Part model, mm, in its own coordinate system. Face numbers are marked on the shaded views. A direction names the side the tool comes from. Round coordinates to 2 decimals unless told otherwise and drop trailing zeros. Write each loop counter-clockwise with the first axis right and the second up, starting at its lowest first coordinate (ties: lowest second). Pieces come first, ordered by that corner, then holes. Notation, with made-up numbers: M 9.5,-0.5 L 48.5,-0.5 A12 cw 48.5,10.5 Z; hole C -22.5,81 d1. An arc over 180 degrees is marked long. Answer as a JSON object with one key per item and string values. Group by question number.
1. Drop flat-ended pins along their axis: pin 1 (12.5 mm diameter, centred on x = -46.71, z = 21.65, fed in from +Y); pin 2 (5 mm diameter, centred on y = -10.5, z = 29.5, fed in from +X); pin 3 (12.5 mm diameter, centred on x = 38.5, y = -14, fed in from +Z); pin 4 (1 mm diameter, centred on x = -34.5, z = 20, fed in from +Y). Give the stop position or say it passes through.
2. Which spindle directions (+Z, -Z, +X, -X, +Y, -Y) get a long thin tool onto all of the face, cutting with end or side? Do the marked faces 4 and 5. Say none if no direction does.
3. Two-plate mould, pull along Z, no slides. Class the marked faces 1, 2 and 3: +Z half, -Z half, draft (parallel to the pull), parting line (faces both ways), or undercut.
4. Band-saw the part on B-B, the plane x = -39. Write the cut outline in (y, z).
5. Band-saw the part on A-A, the plane z = 31. Write the cut outline in (x, y).
6. Band-saw the part on C-C, the plane y = -3. Write the cut outline in (x, z).
7. Band-saw the part on D-D, the plane x = 38. Write the cut outline in (y, z), plus the area to 3 significant figures.
8. Drill centre lines: line 1 (X direction, y = -8.75, z = 13); line 2 (X direction, y = -9.25, z = 15.5); line 3 (X direction, y = -4.5, z = 34). Where is each one in solid material? Low to high. Write a range as from..to.
from build123d import *

# Parameters (mm, degrees)
F0_R     = 10.5768156475
F1_DEPTH = 25.4
F2_R     = 5.8673814398
F3_DEPTH = 32.9165069776
F5_R     = 2.8308188493
F6_DEPTH = 16.9651473331


# Not quite as in the source:
# - a feature names something its author has since deleted; it is built from what else it names


with BuildPart() as f1:
    # F0 (on Front) → F1 (new body)
    with BuildSketch(Plane.XZ):
        Polygon((0, 38.612421602), (-61.9064718485, 38.612421602), (-61.9064718485, 5.6969146244), (1.8989704549, 5.6969146244), (65.7044127584, 12.2800152749), (65.7044127584, 22.1546681132), (65.7044127584, 22.6610619575), (0, 22.6610619575), align=None)
        with Locations((-46.7147007585, 21.6482765973)):
            Circle(F0_R, mode=Mode.SUBTRACT)
    extrude(amount=F1_DEPTH)

    # F2 (on face) → F3 (cut, through all)
    with BuildSketch(Plane.XY.offset(38.612421602)):
        with Locations((-18.1035287678, -13.1292007864)):
            Circle(F2_R)
    extrude(amount=-F3_DEPTH, mode=Mode.SUBTRACT)

    # F5 (on face) → F6 (cut, through all)
    with BuildSketch(Plane.XY.offset(22.6610619575)):
        with Locations((55.3233735263, -12.2800152749)):
            Circle(F5_R)
    extrude(amount=-F6_DEPTH, mode=Mode.SUBTRACT)


solid = f1.part
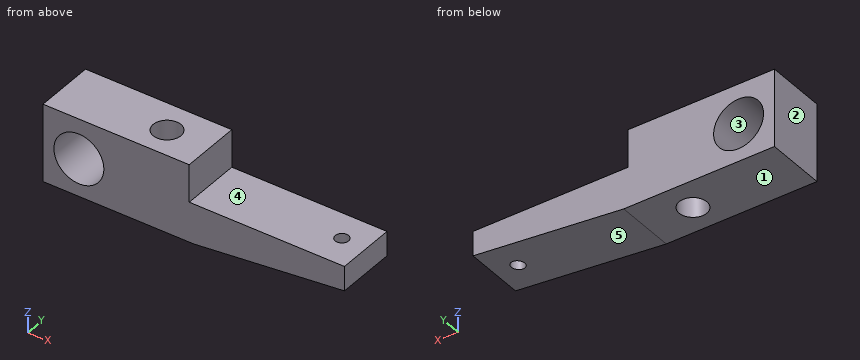
Worked answers:
{
 "1": {"pin 1": "passes through", "pin 2": "stops at x = 0", "pin 3": "stops at z = 22.66", "pin 4": "stops at y = 0"},
 "2": {"face 4": "+Z, +X, +Y, -Y", "face 5": "-Z, +X, +Y, -Y"},
 "3": {"face 1": "-Z half", "face 2": "draft", "face 3": "undercut"},
 "4": {"outline": "M -25.4,5.7 L 0,5.7 L 0,14.41 L -25.4,14.41 Z; M -25.4,28.88 L 0,28.88 L 0,38.61 L -25.4,38.61 Z"},
 "5": {"outline": "M -61.91,-25.4 L -51.66,-25.4 L -51.66,0 L -61.91,0 Z; M -41.77,-25.4 L 0,-25.4 L 0,0 L -41.77,0 Z; hole C -18.1,-13.13 d11.73"},
 "6": {"outline": "M -61.91,5.7 L 1.9,5.7 L 65.7,12.28 L 65.7,22.66 L 0,22.66 L 0,38.61 L -61.91,38.61 Z; hole C -46.71,21.65 d21.15"},
 "7": {"outline": "M -25.4,9.42 L 0,9.42 L 0,22.66 L -25.4,22.66 Z", "area": "336 mm^2"},
 "8": {"line 1": "x = -61.91..-52.8, -40.63..-22.01, -14.2..65.7", "line 2": "x = -61.91..-55.32, -38.11..-22.51, -13.7..65.7", "line 3": "x = -61.91..0"}
}
